Here's the drawing with two shaded views (mm, measured from the low corner). I have some questions. Round coordinates to 2 decimals unless told otherwise and drop trailing zeros. Loops run counter-clockwise (first coordinate to the right, second up) from the corner with the lowest first, then second, coordinate; pieces in that order, holes last. Notation, with made-up numbers: (-38, 79) -> (5, 79) arc R7 cw to (5, 92) -> close; hole circle Ø8 at (11.5, -24.75). An arc over 180 degrees is marked (long way). Write item = value, one per line.
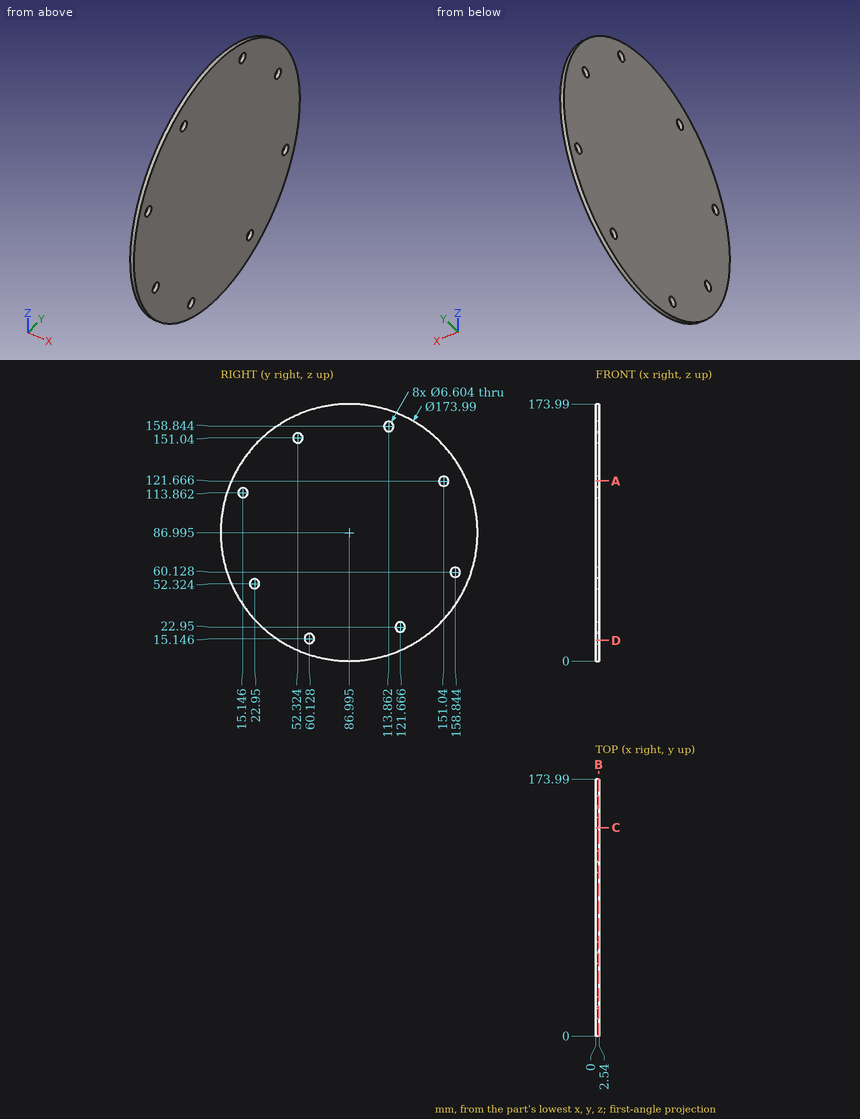
1. I need wall thicknesses on line 1 (Z direction, x = 0.1, y = 20); line 2 (Y direction, x = 1.65, z = 116.5) (1 decimal); line 3 (Z direction, x = 0.7, y = 158.5) (1 decimal). Which ranges of each line are inside material? Lowest first, please. Write a range as [from, to].
Entries:
line_1 = [31.5, 50.84], [53.81, 142.49]
line_2 = [5.2, 13.2], [17.1, 168.8]
line_3 = [37.4, 56.8], [63.4, 136.5]
2. Suppose I cut it at D-D, the plane z = 14. List the corners of the cut face in (x, y) for me (1 decimal).
Entries:
outline = (0, 39.7) -> (2.5, 39.7) -> (2.5, 57) -> (0, 57) -> close; (0, 63.2) -> (2.5, 63.2) -> (2.5, 134.3) -> (0, 134.3) -> close
3. Suppose I cut it at A-A, the plane z = 122. List the corners of the cut face in (x, y) for me (1 decimal).
Entries:
outline = (0, 7.4) -> (2.5, 7.4) -> (2.5, 147.8) -> (0, 147.8) -> close; (0, 154.3) -> (2.5, 154.3) -> (2.5, 166.6) -> (0, 166.6) -> close
4. Suppose I cut it at B-B, the plane x = 2.1. Count the separate pieces of the cut face and the enclosed holes in it, and give its area (3 significant figures).
Entries:
separate_pieces = 1
enclosed_holes = 8
area = 23,500 mm²
5. Suppose I cut it at C-C, the plane y = 141. List the corners of the cut face in (x, z) for me.
Entries:
outline = (0, 18.79) -> (2.54, 18.79) -> (2.54, 155.2) -> (0, 155.2) -> close
6. I'm going to push a flat-ended pin straight in: pin 1 (8.5 mm diameter, centred on y = 60.13, z = 15.15, fed in from -X). Where does the tip first touch, or does it pass through?
Entries:
pin_1 = 0
